Geometry: final body of the model. Coordinates: model frame, mm. A direction names the side the tool comes from. Coordinates: 2 decimals unless noted, no trailing zeros. Order: outer loops, then holes, each group sorted by start corner. A loop starts at its lowest first (then second) coordinate and runs counter-clockwise, first axis right, second up. Notation, with made-up numbers: (-15, -16.5) - (21, -16.5) arc R11 cw to (21, -12.5) - close; hole circle Ø2 at (-23, 47.25). An arc over 180 degrees is marked (long way). Use one line per item in the form item = value. Start each with the question number.
Autodesk Inventor part; units mm, degrees
ref_plane "YZ Plane" through (0, 0, 0) normal (1, 0, 0) x (0, 1, 0)
ref_plane "XZ Plane" through (0, 0, 0) normal (0, 1, 0) x (-1, 0, 0)
ref_plane "XY Plane" through (0, 0, 0) normal (0, 0, 1) x (1, 0, 0)
sketch "Sketch1" plane through (0, 0, 0) normal (0, 0, 1) x (1, 0, 0)
  line L0 (0, 5.25) -> (0, -5.25) construction
  line L1 (-8.75, 0) -> (8.75, 0) construction
  line L2 (-6.25, 3.75) -> (6.25, 3.75)
  line L3 (6.25, 3.75) -> (6.25, -3.75)
  line L4 (6.25, -3.75) -> (-6.25, -3.75)
  line L5 (-6.25, -3.75) -> (-6.25, 3.75)
  point P0 (0, 0)
  dimension "d0" = 7.5
  dimension "d1" = 12.5
extrude "Extrusion1" add sketch "Sketch1" along normal blind 45
sketch "Sketch2" plane through (0, 0, 45) normal (0, 0, 1) x (1, 0, 0)
  line L0 (-6.25, 3.75) -> (6.25, 3.75)
  line L1 (-6.25, -3.75) -> (-6.25, 3.75)
  line L2 (-5, 2.5) -> (5, 2.5)
  line L3 (5, 2.5) -> (5, -2.5)
  line L4 (5, -2.5) -> (-5, -2.5)
  line L5 (-5, -2.5) -> (-5, 2.5)
  point P0 (0, 0)
  dimension "d4" = 10
  dimension "d5" = 5
  dimension "d6" = 1.25
  dimension "d7" = 1.25
extrude "Extrusion2" cut sketch "Sketch2" against normal blind 43.75
properties part number "UQ-203-5x10x45mm" material "Glass"
(1) Draft query along X for faces 3 (the flat face through (6.25, 0, 22)), 4 (the flat face through (0, 3, 45)), 5 (the flat face through (5, 0, 23)). Return one class per face: released by +X, released by -X, zero draft, split by the parting line, or undercut.
(2) Cut plane A-A on z = 38. Return the cut outline in (x, y), plus the area to 4 significant figures.
(3) Set-up query: faces 1 (the flat face through (0, 0, 1.25)), 2 (the flat face through (0, -3.75, 22)). Return all of +Z, -Z, +X, -X, +Y, -Y with unobstructed straight access to the full face (end or side cutting, diameter ignored); none if empty.
(4) Cut plane C-C on y = 2. Return the cut outline in (x, z).
(5) Contact query for flat-ended pins moving along their axis: pin 1 Ø4 at (x, y) = (0, -1) entering from +Z; pin 2 Ø1 at (x, y) = (1.5, -0.5) entering from +Z. Output: stop coordinate, or through.
(6) Cut plane B-B on x = -3.75. Return the cut outline in (y, z).
(7) Material intervals for L1, parallel to Y at x = -1.5, z = 22; L2, parallel to X at y = 1.25, z = 26; L3, parallel to Z at x = -3.5, y = 2, sorted ascending. Write a range as from..to.
Check sheet entries:
q1.face_3 = released by +X
q1.face_4 = zero draft
q1.face_5 = undercut
q2.outline = (-6.25, -3.75) - (6.25, -3.75) - (6.25, 3.75) - (-6.25, 3.75) - close; hole (-5, -2.5) - (5, -2.5) - (5, 2.5) - (-5, 2.5) - close
q2.area = 43.75 mm^2
q3.face_1 = +Z
q3.face_2 = +Z, -Z, +X, -X, -Y
q4.outline = (-6.25, 0) - (6.25, 0) - (6.25, 45) - (5, 45) - (5, 1.25) - (-5, 1.25) - (-5, 45) - (-6.25, 45) - close
q5.pin_1 = 45
q5.pin_2 = 1.25
q6.outline = (-3.75, 0) - (3.75, 0) - (3.75, 45) - (2.5, 45) - (2.5, 1.25) - (-2.5, 1.25) - (-2.5, 45) - (-3.75, 45) - close
q7.L1 = -3.75..-2.5, 2.5..3.75
q7.L2 = -6.25..-5, 5..6.25
q7.L3 = 0..1.25
